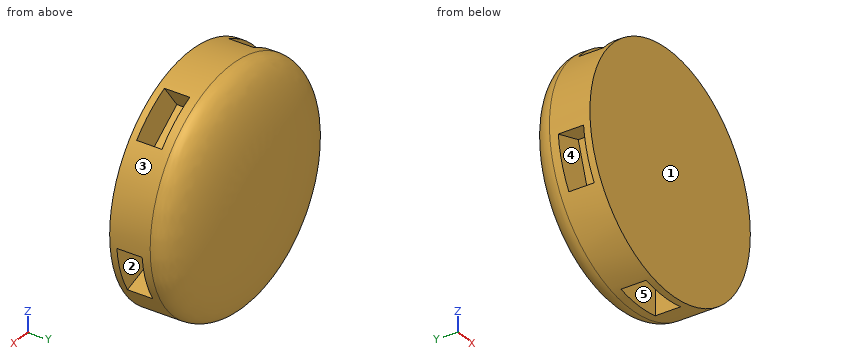
```python
from build123d import *

# Parameters (mm, degrees)
ESQUISSE3_W             = 15
ESQUISSE3_H             = 20
ENL_V_MAT_EXTRU_1_DEPTH = 7.5
ESQUISSE4_R             = 35
BOSS_EXTRU_1_DEPTH      = 2


with BuildPart() as part:
    # Esquisse2 → Révolution1 (revolve)
    with BuildSketch(Plane.XY):
        with BuildLine():
            Line((0, 20), (0, 0))
            Line((0, 0), (35, 0))
            Line((35, 0), (35, 10))
            add(Edge.make_bspline(
                [(0, 20), (32.349399846, 20), (34.80179319, 13.431096766), (35, 10)],
                knots=[0, 0, 0, 0, 1, 1, 1, 1], degree=3))
        make_face()
    revolve(axis=Axis((0, 20, 0), (0, -1, 0)))

    # Esquisse3 → Enlèv. mat.-Extru.1 (cut)
    with BuildSketch(Plane.XZ):
        with Locations((0, -35)):
            Rectangle(ESQUISSE3_W, ESQUISSE3_H)
        Polygon((-45.115170691, -6.772840875), (-26.094040365, -0.592500987), (-21.45878545, -14.858348732), (-40.479915775, -21.038688619), align=None)
        Polygon((-20.382708895, 40.814154139), (-8.627003849, 24.633814252), (-20.762258765, 15.817035467), (-32.517963811, 31.997375355), align=None)
        Polygon((32.517963811, 31.997375355), (20.762258765, 15.817035467), (8.627003849, 24.633814252), (20.382708895, 40.814154139), align=None)
        Polygon((40.479915775, -21.038688619), (21.45878545, -14.858348732), (26.094040365, -0.592500987), (45.115170691, -6.772840875), align=None)
    extrude(amount=-ENL_V_MAT_EXTRU_1_DEPTH, mode=Mode.SUBTRACT)

    # Esquisse4 → Boss.-Extru.1 (add)
    with BuildSketch(Plane.XZ):
        Circle(ESQUISSE4_R)
    extrude(amount=BOSS_EXTRU_1_DEPTH)


solid = part.part
```
For this review, take the finished solid that the model builds, in its own axes (mm). Face numbers are marked on the shaded views. A direction names the side the tool comes from. Coordinates: 2 decimals unless noted, no trailing zeros. Loops run counter-clockwise (first coordinate to the right, second up) from the corner with the lowest first, then second, coordinate; pieces in that order, holes last. Notation, with made-up numbers: (4.5, 24) - (38.5, 24) arc R10 ccw to (38.5, 38) - close; hole circle Ø9 at (78.25, 30.25). An arc over 180 degrees is marked (long way). Use one line per item in the form item = value. Start each with the question number.
1) Take a section at A-A (y = 1.75). State the section outline as (x, z) points, plus the area to 3 significant figures.
2) For the marked faces 1 and 2, list the 3-axis set-ups (+Z, -Z, +X, -X, +Y, -Y) from which the entire face can be reached by the end or side of a thin tool; tool diameter is ignored.
3) Draft analysis for pull direction Z (two halves, no side actions). For the marked faces 3, 4 and 5, state which applies: released by +Z, released by -Z, zero draft, split by the parting line, or undercut.
4) To check wall thickness, follow probe 1 along X at (y, z) = (7.25, 22); probe 2 along Y at (x, z) = (-29, -7); probe 3 along Y at (x, z) = (14, 27). State the ranges of each line that lie inside material, in increasing order. Write a range as from..to.
5) For pin 1 (8 mm diameter, centred on x = -3, y = 4, fed in from -Z); pin 2 (2 mm diameter, centred on y = 3.5, z = -30.5, fed in from -X); pin 3 (8 mm diameter, centred on x = -14, y = 17.5, fed in from +Z), all flat-tipped, find the tip position at first contact; note any pin that passes through.
From the geometry:
q1.outline = (-34.83, -3.43) - (-26.09, -0.59) - (-21.46, -14.86) - (-30.2, -17.7) arc R35 ccw to (-7.5, -34.19) - (-7.5, -25) - (7.5, -25) - (7.5, -34.19) arc R35 ccw to (30.2, -17.7) - (21.46, -14.86) - (26.09, -0.59) - (34.83, -3.43) arc R35 ccw to (26.16, 23.25) - (20.76, 15.82) - (8.63, 24.63) - (14.03, 32.07) arc R35 ccw to (-14.03, 32.07) - (-8.63, 24.63) - (-20.76, 15.82) - (-26.16, 23.25) arc R35 ccw to start
q1.area = 3,120 mm2
q2.face_1 = +Z, -Z, +X, -X, -Y
q2.face_2 = none
q3.face_3 = split by the parting line
q3.face_4 = undercut
q3.face_5 = zero draft
q4.probe_1 = -27.22..-25.25, -12.25..12.25, 25.25..27.22
q4.probe_2 = -2..0, 7.5..16.16
q4.probe_3 = -2..0, 7.5..15.88
q5.pin_1 = -34.98
q5.pin_2 = -18.83
q5.pin_3 = 30.93
